Can you work these out from the model? Positions are in its coordinate system, mm. A direction names the side the tool comes from. Round coordinates to 2 decimals unless told otherwise and drop trailing zeros. Loops run counter-clockwise (first coordinate to the right, second up) from the corner with the lowest first, then second, coordinate; pieces in that order, holes last.
(1) Will these pins go through, and if not, where does the flat tip stop? pin 1 Ø1.5 at (x, z) = (47, 1.5) entering from -Y; pin 2 Ø0.9 at (x, z) = (-46.5, 1.5) entering from +Y.
(2) Which directions (+Z, -Z, +X, -X, +Y, -Y) give clear straight access to the entire face, cutting with the end or side of a thin tool? Please do faces 5 (the face through (45, -37, 1)), 6 (the face through (-35, 38, 1)), 7 (the face through (-60, -40, 1)), 8 (the face through (22, -5, 1)).
(3) I want a section at C-C on z = 2.5. Give the number of separate pieces and of enclosed holes in the cut face, plus the area to 3 significant figures.
(4) If I drill on line 1 along X through (y, z) = (-4, 2.65); line 2 along Y through (x, z) = (15.5, 1.75); line 3 along Y through (x, z) = (35.5, 2), over which ranges is the centre line in solid material (lowest first)?
(5) I want a section at A-A on x = -57. Write out the boundary of the cut face in (y, z), plus the area to 3 significant figures.
(6) Thinking about a two-plate mould opening in Y: for faces 1 (the face through (-55, -38, 1)), 2 (the face through (-32.75, 9.04, 1.48)), 3 (the face through (60, -40, 1)), 4 (the face through (0, 40, 1)), which applies, released by +Y, released by -Y, zero draft, split by the parting line, or undercut?
(7) I want a section at B-B on y = -9. Write out the boundary of the cut face in (x, z).
from build123d import *

# Parameters (mm, degrees)
SKETCH1_R           = 1.5
SKETCH1_W           = 3
SKETCH1_H           = 10
BOSS_EXTRUDE1_DEPTH = 3
SKETCH2_W           = 10
SKETCH2_H           = 3
CUT_EXTRUDE2_DEPTH  = 3


with BuildPart() as part:
    # Sketch1 → Boss-Extrude1 (new body)
    with BuildSketch(Plane.XY):
        Polygon((-55, 40), (-55, 37), (-35, 37), (-35, 40), (35, 40), (35, 37), (55, 37), (55, 40), (65, 40), (65, -40), (55, -40), (55, -37), (35, -37), (35, -40), (-35, -40), (-35, -37), (-55, -37), (-55, -40), (-65, -40), (-65, 40), align=None)
        with Locations((15.5, 15.5)):
            Circle(SKETCH1_R, mode=Mode.SUBTRACT)
        with Locations((-15.5, 15.5)):
            Circle(SKETCH1_R, mode=Mode.SUBTRACT)
        with Locations((15.5, -15.5)):
            Circle(SKETCH1_R, mode=Mode.SUBTRACT)
        with Locations((-15.5, -15.5)):
            Circle(SKETCH1_R, mode=Mode.SUBTRACT)
        with Locations((22.5, 0)):
            Rectangle(SKETCH1_W, SKETCH1_H, mode=Mode.SUBTRACT)
        with Locations((-22.5, 0)):
            Rectangle(SKETCH1_W, SKETCH1_H, mode=Mode.SUBTRACT)
        with BuildLine():
            Line((-60.75, 11), (-34.75, 11))
            ThreePointArc((-34.75, 11), (-32.75, 9), (-34.75, 7))
            Line((-34.75, 7), (-60.75, 7))
            ThreePointArc((-60.75, 7), (-62.75, 9), (-60.75, 11))
        make_face(mode=Mode.SUBTRACT)
        with BuildLine():
            Line((-34.75, -7), (-60.75, -7))
            ThreePointArc((-60.75, -7), (-62.75, -9), (-60.75, -11))
            Line((-60.75, -11), (-34.75, -11))
            ThreePointArc((-34.75, -11), (-32.75, -9), (-34.75, -7))
        make_face(mode=Mode.SUBTRACT)
        with BuildLine():
            Line((34.75, 11), (60.75, 11))
            ThreePointArc((60.75, 11), (62.75, 9), (60.75, 7))
            Line((60.75, 7), (34.75, 7))
            ThreePointArc((34.75, 7), (32.75, 9), (34.75, 11))
        make_face(mode=Mode.SUBTRACT)
        with BuildLine():
            Line((34.75, -7), (60.75, -7))
            ThreePointArc((60.75, -7), (62.75, -9), (60.75, -11))
            Line((60.75, -11), (34.75, -11))
            ThreePointArc((34.75, -11), (32.75, -9), (34.75, -7))
        make_face(mode=Mode.SUBTRACT)
    extrude(amount=BOSS_EXTRUDE1_DEPTH)

    # Sketch2 → Cut-Extrude2 (cut)
    with BuildSketch(Plane.XY.offset(3)):
        with Locations((0, 3.25)):
            Rectangle(SKETCH2_W, SKETCH2_H)
        with Locations((0, -3.25)):
            Rectangle(SKETCH2_W, SKETCH2_H)
    extrude(amount=-CUT_EXTRUDE2_DEPTH, mode=Mode.SUBTRACT)


solid = part.part
Filled sheet:
1. pin 1: stops at y = -37
1. pin 2: stops at y = 37
2. face 5: +Z, -Z, -Y
2. face 6: +Z, -Z, +Y
2. face 7: +Z, -Z, +X, -X, -Y
2. face 8: +Z, -Z
3. separate pieces: 1
3. enclosed holes: 12
3. area: 9,550 mm2
4. line 1: x = -65 to -24, -21 to -5, 5 to 21, 24 to 65
4. line 2: y = -40 to -17, -14 to 14, 17 to 40
4. line 3: y = -37 to -11, -7 to 7, 11 to 37
5. outline: (-40, 0) - (-11, 0) - (-11, 3) - (-40, 3) - close; (-7, 0) - (7, 0) - (7, 3) - (-7, 3) - close; (11, 0) - (40, 0) - (40, 3) - (11, 3) - close
5. area: 216 mm2
6. face 1: zero draft
6. face 2: undercut
6. face 3: released by -Y
6. face 4: released by +Y
7. outline: (-65, 0) - (-62.75, 0) - (-62.75, 3) - (-65, 3) - close; (-32.75, 0) - (32.75, 0) - (32.75, 3) - (-32.75, 3) - close; (62.75, 0) - (65, 0) - (65, 3) - (62.75, 3) - close
